```python
from build123d import *

# Parameters (mm, degrees)
IZIM4_R                          = 3.75
IZIM4_R_2                        = 1.75
Y_KSEKLIK_EKSTR_ZYON1_DEPTH      = 5
IZIM5_R                          = 2.1
KES_EKSTR_ZYON1_DEPTH            = 24
KES_EKSTR_ZYON2_DEPTH            = 36.170331308
Y_KSEKLIK_EKSTR_ZYON2_REACH      = 67.295
Y_KSEKLIK_EKSTR_ZYON2_END_RADIUS = 20
Y_KSEKLIK_EKSTR_ZYON2_START      = -5
DAIRESEL_KAPLAMA1_COUNT          = 3
KES_EKSTR_ZYON3_DEPTH            = 45
KES_EKSTR_ZYON3_DEPTH_BACK       = 39
IZIM10_W                         = 61.268894521
IZIM10_H                         = 17.891205564


with BuildPart() as part:
    # Çizim3 → Döndür1 (revolve)
    with BuildSketch(Plane.XY, mode=Mode.PRIVATE) as d_nd_r1_sk:
        with BuildLine():
            Line((-11.490666647, -9.641814145), (-15.320888862, -12.855752194))
            ThreePointArc((-15.320888862, -12.855752194), (-18.793852416, -6.840402867), (-20, 0))
            Line((-20, 0), (-15, 0))
            ThreePointArc((-15, 0), (-14.095389312, -5.13030215), (-11.490666647, -9.641814145))
        make_face()
    revolve(d_nd_r1_sk.sketch.rotate(Axis((0, 24.311963794, 0), (0, -1, 0)), 270), axis=Axis((0, 24.311963794, 0), (0, -1, 0)))

    # Çizim4 → Yükseklik-Ekstrüzyon1 (add)
    # profile 1 of 3: a face of its own
    with BuildSketch(Plane(origin=(0, 0, 0), x_dir=(1, 0, 0), z_dir=(0, 1, 0))):
        with Locations((10, 17.320508076)):
            Circle(IZIM4_R)
        with Locations((10, 17.320508076)):
            Circle(IZIM4_R_2, mode=Mode.SUBTRACT)
    # profile 2 of 3: a face of its own
    with BuildSketch(Plane(origin=(0, 0, 0), x_dir=(1, 0, 0), z_dir=(0, 1, 0))):
        with Locations((-20, 0)):
            Circle(IZIM4_R)
        with Locations((-20, 0)):
            Circle(IZIM4_R_2, mode=Mode.SUBTRACT)
    # profile 3 of 3: a face of its own
    with BuildSketch(Plane(origin=(0, 0, 0), x_dir=(1, 0, 0), z_dir=(0, 1, 0))):
        with Locations((10, -17.320508076)):
            Circle(IZIM4_R)
        with Locations((10, -17.320508076)):
            Circle(IZIM4_R_2, mode=Mode.SUBTRACT)
    extrude(amount=-Y_KSEKLIK_EKSTR_ZYON1_DEPTH)

    # Çizim5 → Kes-Ekstrüzyon1 (cut)
    with BuildSketch(Plane(origin=(0, 0, 0), x_dir=(1, 0, 0), z_dir=(0, 1, 0))):
        with Locations(Location((10, 17.320508076, 0), (0, 0, 270))):
            Circle(IZIM5_R)
        with Locations(Location((-20, 0, 0), (0, 0, 270))):
            Circle(IZIM5_R)
        with Locations(Location((10, -17.320508076, 0), (0, 0, 270))):
            Circle(IZIM5_R)
    extrude(amount=-KES_EKSTR_ZYON1_DEPTH, mode=Mode.SUBTRACT)

    # Çizim6 → Kes-Ekstrüzyon2 (cut)
    with BuildSketch(Plane(origin=(0, -41.170331308, 0), x_dir=(1, 0, 0), z_dir=(0, 1, 0))):
        Polygon((-16, 0), (-18, 3.464101615), (-22, 3.464101615), (-24, 0), (-22, -3.464101615), (-18, -3.464101615), align=None)
        Polygon((8.769230769, 14.300522052), (12.769230769, 14.300522052), (14.769230769, 17.764623667), (12.769230769, 21.228725283), (8.769230769, 21.228725283), (6.769230769, 17.764623667), align=None)
        Polygon((8.769230769, -14.300522052), (6.769230769, -17.764623667), (8.769230769, -21.228725283), (12.769230769, -21.228725283), (14.769230769, -17.764623667), (12.769230769, -14.300522052), align=None)
    extrude(amount=KES_EKSTR_ZYON2_DEPTH, mode=Mode.SUBTRACT)

    # Yükseklik-Ekstrüzyon2: up to this sphere (the profile starts outside it)
    y_kseklik_ekstr_zyon2_end = Location((0, 0, 0)) * Sphere(Y_KSEKLIK_EKSTR_ZYON2_END_RADIUS, mode=Mode.PRIVATE)
    # Çizim9 → Yükseklik-Ekstrüzyon2 (add, up to the surface)
    with BuildSketch(Plane(origin=(26.738833579, -25.345051489, 0), x_dir=(-0.8746197071393953, -0.48480962024633817, 0), z_dir=(0.48480962024633817, -0.8746197071393953, 0)).offset(Y_KSEKLIK_EKSTR_ZYON2_START), mode=Mode.PRIVATE) as y_kseklik_ekstr_zyon2_sk1:
        Polygon((3.967200538, 6.871392896), (-3.967200538, 6.871392896), (-7.934401077, 0), (-3.967200538, -6.871392896), (3.967200538, -6.871392896), (7.934401077, 0), align=None)
        Polygon((5.625, 0), (2.8125, 4.871392896), (-2.8125, 4.871392896), (-5.625, 0), (-2.8125, -4.871392896), (2.8125, -4.871392896), align=None, mode=Mode.SUBTRACT)
    y_kseklik_ekstr_zyon2_tool1 = extrude(y_kseklik_ekstr_zyon2_sk1.sketch, amount=-Y_KSEKLIK_EKSTR_ZYON2_REACH, mode=Mode.PRIVATE) - y_kseklik_ekstr_zyon2_end
    y_kseklik_ekstr_zyon2 = y_kseklik_ekstr_zyon2_tool1.solids().sort_by_distance((24.314785, -20.971953, -6.661468))[0]
    add(y_kseklik_ekstr_zyon2)

    # Dairesel Kaplama1: Yükseklik-Ekstrüzyon2 ×3 about axis
    dairesel_kaplama1_axis = Axis((0, 0, 0), (0, 1, 0))
    for i in range(1, DAIRESEL_KAPLAMA1_COUNT):
        add(y_kseklik_ekstr_zyon2.rotate(dairesel_kaplama1_axis, i * 360 / DAIRESEL_KAPLAMA1_COUNT))

    # Çizim10 → Kes-Ekstrüzyon3 (cut, two sides: drawn at the far end of the back side and taken through both)
    with BuildSketch(Plane.XY.offset(-KES_EKSTR_ZYON3_DEPTH_BACK)):
        with Locations((5.148097131, 8.945602782)):
            Rectangle(IZIM10_W, IZIM10_H)
    extrude(amount=KES_EKSTR_ZYON3_DEPTH + KES_EKSTR_ZYON3_DEPTH_BACK, mode=Mode.SUBTRACT)


solid = part.part
```
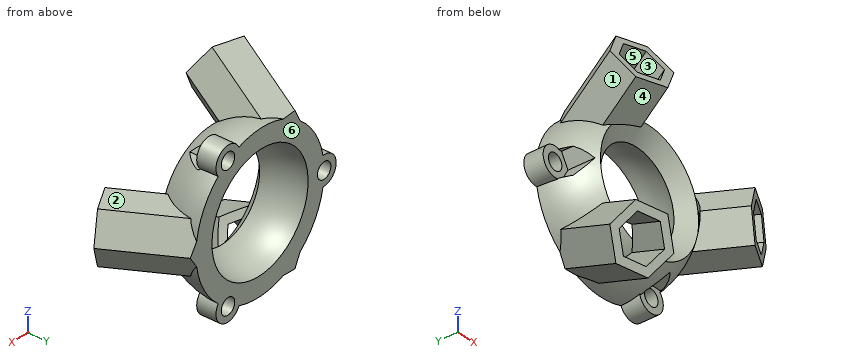
Check sheet for the modelled part. Datum: model origin and axes. Units: mm. Face numbers are marked on the shaded views. A direction names the side the tool comes from. Round coordinates to 2 decimals unless told otherwise and drop trailing zeros. Order: outer loops, then holes, each group sorted by start corner. A loop starts at its lowest first (then second) coordinate and runs counter-clockwise, first axis right, second up. Notation, with made-up numbers: M 45.25,18 L 57.25,18 A22 ccw 57.25,57 Z; hole C -36,51.25 d8. An arc over 180 degrees is marked long. Answer in a Markdown table with one row per item.
(1) Section check C-C on x = 10. Give the number of separate pieces and of enclosed holes in the cut face, plus the area to 3 significant figures.
Findings:
| item | result |
|---|---|
| separate pieces | 4 |
| enclosed holes | 0 |
| area | 144 mm^2 |
(2) Section check A-A on x = 0. Record the boundary of the cut face in (y, z), plus the area to 3 significant figures.
Findings:
| item | result |
|---|---|
| outline | M -12.86,-15.32 A20 ccw 0,-20 L 0,-15 A15 cw -9.64,-11.49 Z; M -12.86,15.32 L -9.64,11.49 A15 cw 0,15 L 0,20 A20 ccw Z |
| area | 122 mm^2 |
(3) Material ranges on line 1 along Z through (x, y) = (21, -12.25); line 2 along X through (y, z) = (-8.5, -4); line 3 along Z through (x, y) = (-20, -2.3), recorded low to high. Write a range as from..to.
Findings:
| item | result |
|---|---|
| line 1 | z = -6.87..-4.87, 4.87..6.87 |
| line 2 | x = -17.66..-11.69, 11.69..17.66, 21.19..23.83 |
| line 3 | z = -3.75..-2.1, 2.1..3.75 |
(4) Set-up check for the marked faces 4, 5 and 6: record each of +Z, -Z, +X, -X, +Y, -Y from which the full face is reachable in a straight line by a thin tool's end or side.
Findings:
| item | result |
|---|---|
| face 4 | -X, -Y |
| face 5 | none |
| face 6 | +Z, -Z, +X, -X, +Y |
(5) Section check B-B on x = 25. Record the boundary of the cut face in (y, z).
Findings:
| item | result |
|---|---|
| outline | M -20.59,-6.87 L -14.03,-6.87 L -5.84,0 L -14.03,6.87 L -20.59,6.87 L -20.59,4.87 L -16.41,4.87 L -10.61,0 L -16.41,-4.87 L -20.59,-4.87 Z |
(6) Gauge pin test, flat ends, axial feed: pin 1 (7.5 mm diameter, centred on x = 11, z = -17.5, fed in from -Y); pin 2 (2 mm diameter, centred on x = 10.5, y = -7, fed in from -Z); pin 3 (1.5 mm diameter, centred on y = -5, z = -9, fed in from +X) (3 decimals); pin 4 (3 mm diameter, centred on x = 8.5, z = -4, fed in from +Y). Record the tip position at first contact, or that the pin passes through.
Findings:
| item | result |
|---|---|
| pin 1 | stops at y = -10.66 |
| pin 2 | stops at z = -14.3 |
| pin 3 | stops at x = 17.575 |
| pin 4 | passes through |
(7) Draft check along X on the marked faces 1, 2 and 3. Enter one of: +X half, -X half, draft (parallel to the pull), parting line (faces both ways), or undercut.
Findings:
| item | result |
|---|---|
| face 1 | -X half |
| face 2 | draft |
| face 3 | undercut |
